The drawing under review shows one solid part. Ordinate dimensions are in mm from its lowest x, y, z. A direction names the side the tool comes from. Coordinates: 2 decimals unless noted, no trailing zeros. Loops run counter-clockwise (first coordinate to the right, second up) from the corner with the lowest first, then second, coordinate; pieces in that order, holes last. Notation, with made-up numbers: (39.25, 22.5) - (85.25, 22.5) arc R5 cw to (85.25, 27.5) - close; hole circle Ø6 at (74, 14). An arc over 180 degrees is marked (long way). Use one line per item in the form item = value. Start each with the question number.
1. For pin 1 Ø1 at (y, z) = (10.5, 7.5) entering from +X; pin 2 Ø8 at (y, z) = (6, 8) entering from +X; pin 3 Ø5 at (x, z) = (11.5, 6) entering from -Y, all flat-tipped, find the tip position at first contact; note any pin that passes through.
2. Draft analysis for pull direction X (two halves, no side actions). For the marked faces 3, 4 and 5, state which applies: +X half, -X half, draft (parallel to the pull), parting line (faces both ways), or undercut.
3. Machinability: for the marked faces 1 and 2, which of the approach directions +Z, -Z, +X, -X, +Y, -Y give a long, thin tool a straight path to every point of the face, cutting with its end or side? Answer none if there is none.
4. To check wall thickness, follow probe 1 along X at (y, z) = (9.5, 13.5) (1 decimal); probe 2 along Y at (x, z) = (7.5, 1); probe 3 along Y at (x, z) = (8.5, 3) (1 decimal). State the ranges of each line that lie inside material, in increasing order.
5. Add section B-B on x = 8. Give the boundary of the cut face in (y, z) (1 decimal).
6. Add section A-A on y = 6.5. Give the boundary of the cut face in (x, z).
7. Add section C-C on y = 3.25. Give the boundary of the cut face in (x, z) (1 decimal).
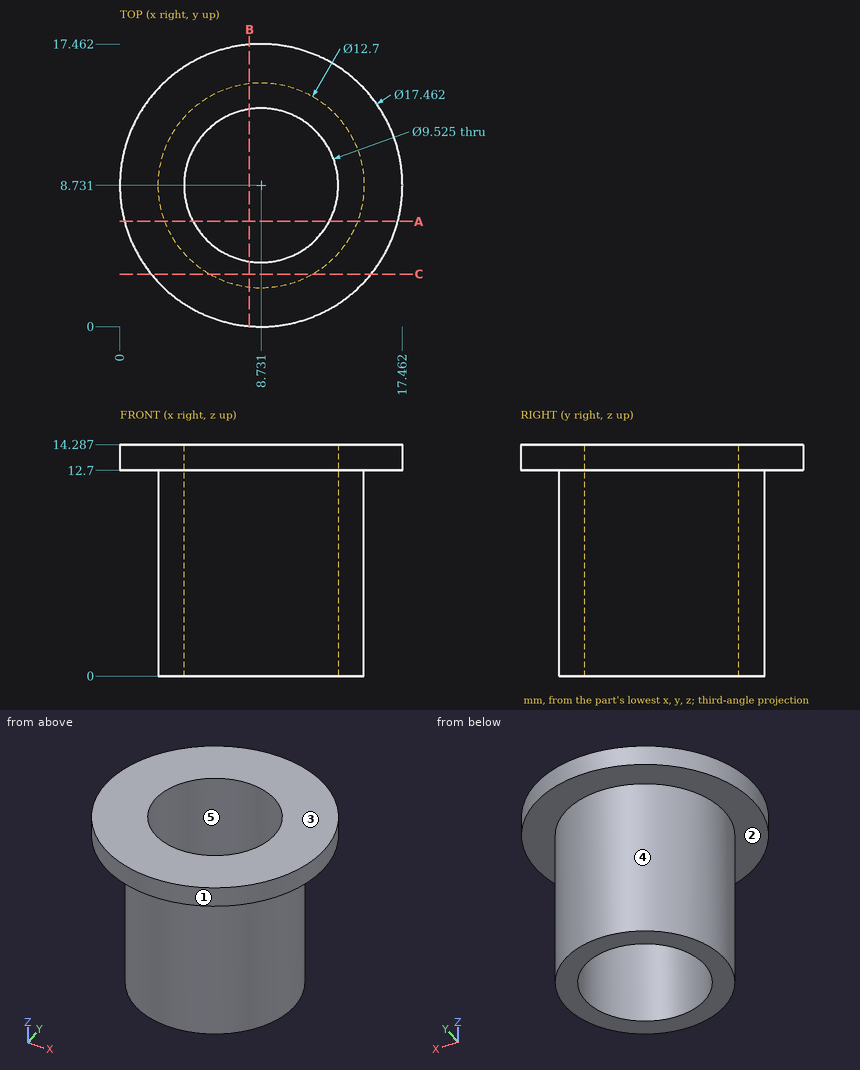
Conclusion:
q1.pin_1 = 14.95
q1.pin_2 = 15.08
q1.pin_3 = 2.39
q2.face_3 = draft
q2.face_4 = parting line
q2.face_5 = undercut
q3.face_1 = +Z, -Z
q3.face_2 = -Z
q4.probe_1 = 0 to 4, 13.4 to 17.4
q4.probe_2 = 2.5 to 4.13, 13.33 to 14.96
q4.probe_3 = 2.4 to 4, 13.5 to 15.1
q5.outline = (0, 12.7) - (2.4, 12.7) - (2.4, 0) - (4, 0) - (4, 14.3) - (0, 14.3) - close; (13.4, 0) - (15, 0) - (15, 12.7) - (17.4, 12.7) - (17.4, 14.3) - (13.4, 14.3) - close
q6.outline = (0.29, 12.7) - (2.79, 12.7) - (2.79, 0) - (4.52, 0) - (4.52, 14.29) - (0.29, 14.29) - close; (12.94, 0) - (14.68, 0) - (14.68, 12.7) - (17.17, 12.7) - (17.17, 14.29) - (12.94, 14.29) - close
q7.outline = (1.9, 12.7) - (5.5, 12.7) - (5.5, 0) - (11.9, 0) - (11.9, 12.7) - (15.5, 12.7) - (15.5, 14.3) - (1.9, 14.3) - close
